Source: CAD feature listing. Evaluate the final solid. Frame: model axes, mm. Coordinates: 2 decimals unless noted, no trailing zeros. Write each loop counter-clockwise with the first axis right and the second up, starting at its lowest first coordinate (ties: lowest second). Pieces come first, ordered by that corner, then holes. Notation, with made-up numbers: (-35.5, 55) - (1.5, 55) arc R16 cw to (1.5, 81) - close; hole circle Ø8 at (-28, -37.75). An arc over 180 degrees is marked (long way). One line per item, written item: value.
from build123d import *

# Parameters (mm, degrees)
EXTRUDE_1_DEPTH     = 2
SKETCH_2_W          = 92
SKETCH_2_H          = 50
CUT_EXTRUDE_1_DEPTH = 87.787095815


with BuildPart() as part:
    # Эскиз1 → Бобышка-Вытянуть1 (new body)
    with BuildSketch(Plane.XY):
        with BuildLine():
            Line((-40, 38), (40, 38))
            ThreePointArc((40, 38), (78, 0), (40, -38))
            Line((40, -38), (-40, -38))
            ThreePointArc((-40, -38), (-78, 0), (-40, 38))
        make_face()
    extrude(amount=EXTRUDE_1_DEPTH)

    # Эскиз2 → Вырез-Вытянуть1 (cut, through all)
    with BuildSketch(Plane.XY.offset(2)):
        Rectangle(SKETCH_2_W, SKETCH_2_H)
    extrude(amount=-CUT_EXTRUDE_1_DEPTH, mode=Mode.SUBTRACT)


solid = part.part
1) Section query C-C on y = -8.5. Output: boundary loops of the cut face in (x, z).
Values found:
outline: (-77.04, 0) - (-46, 0) - (-46, 2) - (-77.04, 2) - close; (46, 0) - (77.04, 0) - (77.04, 2) - (46, 2) - close
2) Section query D-D on x = 55. Output: boundary loops of the cut face in (y, z), then the cut area to 3 significant figures.
Values found:
outline: (-34.91, 0) - (34.91, 0) - (34.91, 2) - (-34.91, 2) - close
area: 140 mm2
3) Section query B-B on z = 1.7. Output: boundary loops of the cut face in (x, y).
Values found:
outline: (-40, -38) - (40, -38) arc R38 ccw to (40, 38) - (-40, 38) arc R38 ccw to start; hole (-46, -25) - (46, -25) - (46, 25) - (-46, 25) - close
4) Contact query for flat-ended pins moving along their axis: P1, Ø1, axis at y = 0, z = 1.5, coming from the -X side; P2, Ø1, axis at y = -30, z = 0.5, coming from the -X side; P3, Ø1, axis at x = -61, y = 11.5, coming from the -Z side. Output: stop coordinate, or through.
Values found:
P1: x = -78
P2: x = -63.95
P3: z = 0
5) Section query A-A on y = 0. Output: boundary loops of the cut face in (x, z).
Values found:
outline: (-78, 0) - (-46, 0) - (-46, 2) - (-78, 2) - close; (46, 0) - (78, 0) - (78, 2) - (46, 2) - close
6) Material intervals for line 1 (Y direction, x = 5, z = 1.05); line 2 (X direction, y = 12, z = 1.7); line 3 (Y direction, x = -45.5, z = 0.8), sorted ascending.
Values found:
line 1: -38 to -25, 25 to 38
line 2: -76.06 to -46, 46 to 76.06
line 3: -37.6 to -25, 25 to 37.6
